Build history of the part. All positions in model axes, mm. Give positions to 0.01 mm unless a question says otherwise; leave off trailing zeros. Write each loop counter-clockwise with the first axis right and the second up, starting at its lowest first coordinate (ties: lowest second). Pieces come first, ordered by that corner, then holes.
from build123d import *

# Parameters (mm, degrees)
SKETCH1_R           = 1.575
SKETCH1_R_2         = 1.5
BOSS_EXTRUDE1_DEPTH = 3
FILLET1_R           = 5
SKETCH2_R           = 1.6
SKETCH2_R_2         = 1.5
SKETCH2_W           = 1
SKETCH2_H           = 3
SKETCH2_W_2         = 1.255583802
CUT_EXTRUDE1_DEPTH  = 3


with BuildPart() as part:
    # Sketch1 → Boss-Extrude1 (new body)
    with BuildSketch(Plane(origin=(0, 0, 0), x_dir=(1, 0, 0), z_dir=(0, 1, 0))):
        Polygon((30.311923219, 82.53968254), (-139.688076781, 82.53968254), (-139.688076781, -117.46031746), (30.311923219, -117.46031746), (30.311923219, -77.46031746), (110.311923219, -77.46031746), (110.311923219, 42.53968254), (30.311923219, 42.53968254), align=None)
        with Locations(Location((-126.688076781, -17.46031746, 0), (0, 0, 270))):
            Circle(SKETCH1_R, mode=Mode.SUBTRACT)
        with Locations(Location((-116.188076781, -11.398139634, 0), (0, 0, 270))):
            Circle(SKETCH1_R, mode=Mode.SUBTRACT)
        with Locations(Location((-116.188076781, -23.522495287, 0), (0, 0, 270))):
            Circle(SKETCH1_R, mode=Mode.SUBTRACT)
        with Locations(Location((-129.688076781, 72.53968254, 0), (0, 0, 270))):
            Circle(SKETCH1_R_2, mode=Mode.SUBTRACT)
        with Locations(Location((20.311923219, 72.53968254, 0), (0, 0, 270))):
            Circle(SKETCH1_R_2, mode=Mode.SUBTRACT)
        with Locations(Location((81.311923219, 35.03968254, 0), (0, 0, 270))):
            Circle(SKETCH1_R_2, mode=Mode.SUBTRACT)
        with Locations(Location((81.311923219, 25.03968254, 0), (0, 0, 270))):
            Circle(SKETCH1_R_2, mode=Mode.SUBTRACT)
        with Locations(Location((81.311923219, 15.03968254, 0), (0, 0, 270))):
            Circle(SKETCH1_R_2, mode=Mode.SUBTRACT)
        with Locations(Location((81.311923219, 5.03968254, 0), (0, 0, 270))):
            Circle(SKETCH1_R_2, mode=Mode.SUBTRACT)
        with Locations(Location((81.311923219, -4.96031746, 0), (0, 0, 270))):
            Circle(SKETCH1_R_2, mode=Mode.SUBTRACT)
        with Locations(Location((59.311923219, -4.96031746, 0), (0, 0, 90))):
            Circle(SKETCH1_R_2, mode=Mode.SUBTRACT)
        with Locations(Location((59.311923219, 5.03968254, 0), (0, 0, 90))):
            Circle(SKETCH1_R_2, mode=Mode.SUBTRACT)
        with Locations(Location((59.311923219, 15.03968254, 0), (0, 0, 90))):
            Circle(SKETCH1_R_2, mode=Mode.SUBTRACT)
        with Locations(Location((59.311923219, 25.03968254, 0), (0, 0, 90))):
            Circle(SKETCH1_R_2, mode=Mode.SUBTRACT)
        with Locations(Location((59.311923219, 35.03968254, 0), (0, 0, 90))):
            Circle(SKETCH1_R_2, mode=Mode.SUBTRACT)
        with Locations(Location((81.311923219, -69.96031746, 0), (0, 0, 90))):
            Circle(SKETCH1_R_2, mode=Mode.SUBTRACT)
        with Locations(Location((81.311923219, -59.96031746, 0), (0, 0, 90))):
            Circle(SKETCH1_R_2, mode=Mode.SUBTRACT)
        with Locations(Location((81.311923219, -49.96031746, 0), (0, 0, 90))):
            Circle(SKETCH1_R_2, mode=Mode.SUBTRACT)
        with Locations(Location((81.311923219, -39.96031746, 0), (0, 0, 90))):
            Circle(SKETCH1_R_2, mode=Mode.SUBTRACT)
        with Locations(Location((81.311923219, -29.96031746, 0), (0, 0, 90))):
            Circle(SKETCH1_R_2, mode=Mode.SUBTRACT)
        with Locations(Location((59.311923219, -29.96031746, 0), (0, 0, 270))):
            Circle(SKETCH1_R_2, mode=Mode.SUBTRACT)
        with Locations(Location((59.311923219, -39.96031746, 0), (0, 0, 270))):
            Circle(SKETCH1_R_2, mode=Mode.SUBTRACT)
        with Locations(Location((59.311923219, -49.96031746, 0), (0, 0, 270))):
            Circle(SKETCH1_R_2, mode=Mode.SUBTRACT)
        with Locations(Location((59.311923219, -59.96031746, 0), (0, 0, 270))):
            Circle(SKETCH1_R_2, mode=Mode.SUBTRACT)
        with Locations(Location((59.311923219, -69.96031746, 0), (0, 0, 270))):
            Circle(SKETCH1_R_2, mode=Mode.SUBTRACT)
        with Locations(Location((100.311923219, 32.53968254, 0), (0, 0, 270))):
            Circle(SKETCH1_R_2, mode=Mode.SUBTRACT)
        with Locations(Location((40.311923219, 32.53968254, 0), (0, 0, 90))):
            Circle(SKETCH1_R_2, mode=Mode.SUBTRACT)
        with Locations(Location((100.311923219, -67.46031746, 0), (0, 0, 90))):
            Circle(SKETCH1_R_2, mode=Mode.SUBTRACT)
        with Locations(Location((40.311923219, -67.46031746, 0), (0, 0, 270))):
            Circle(SKETCH1_R_2, mode=Mode.SUBTRACT)
        with Locations(Location((20.311923219, -107.46031746, 0), (0, 0, 90))):
            Circle(SKETCH1_R_2, mode=Mode.SUBTRACT)
        with Locations(Location((-129.688076781, -107.46031746, 0), (0, 0, 90))):
            Circle(SKETCH1_R_2, mode=Mode.SUBTRACT)
    extrude(amount=BOSS_EXTRUDE1_DEPTH)

    # Fillet1
    fillet1_edges = [part.edges().sort_by_distance(p)[0] for p in [
        (-139.688076781, 1.5, -82.53968254),
        (30.311923219, 1.5, -82.53968254),
        (30.311923219, 1.5, -42.53968254),
        (110.311923219, 1.5, -42.53968254),
        (110.311923219, 1.5, 77.46031746),
        (30.311923219, 1.5, 77.46031746),
        (30.311923219, 1.5, 117.46031746),
        (-139.688076781, 1.5, 117.46031746),
    ]]
    fillet(fillet1_edges, radius=FILLET1_R)

    # Sketch2 → Cut-Extrude1 (cut)
    with BuildSketch(Plane(origin=(0, 3, 0), x_dir=(1, 0, 0), z_dir=(0, 1, 0))):
        with Locations(Location((101.931923219, -39.05031746, 0), (0, 0, 270))):
            Circle(SKETCH2_R)
        with Locations(Location((94.311923219, 4.12968254, 0), (0, 0, 270))):
            Circle(SKETCH2_R)
        with Locations(Location((41.101923219, -7.85531746, 0), (0, 0, 270))):
            Circle(SKETCH2_R)
        with Locations(Location((41.101923219, 11.35468254, 0), (0, 0, 270))):
            Circle(SKETCH2_R)
        with Locations(Location((41.101923219, -46.27531746, 0), (0, 0, 270))):
            Circle(SKETCH2_R)
        with Locations(Location((41.101923219, -27.06531746, 0), (0, 0, 270))):
            Circle(SKETCH2_R)
        with Locations(Location((-14.518076781, -7.85531746, 0), (0, 0, 270))):
            Circle(SKETCH2_R)
        with Locations(Location((-14.518076781, 11.35468254, 0), (0, 0, 270))):
            Circle(SKETCH2_R)
        with Locations(Location((-14.518076781, -27.06531746, 0), (0, 0, 270))):
            Circle(SKETCH2_R)
        with Locations(Location((-14.518076781, -46.27531746, 0), (0, 0, 270))):
            Circle(SKETCH2_R)
        with Locations(Location((-49.062510974, -52.38531746, 0), (0, 0, 270))):
            Circle(SKETCH2_R_2)
        with Locations(Location((-49.062510974, 17.46468254, 0), (0, 0, 270))):
            Circle(SKETCH2_R_2)
        with Locations(Location((70.311923219, -51.21031746, 0), (0, 0, 270))):
            Circle(SKETCH2_R_2)
        with Locations(Location((70.311923219, 16.28968254, 0), (0, 0, 270))):
            Circle(SKETCH2_R_2)
        with Locations(Location((27.931923219, 14.35968254, 0), (0, 0, 270))):
            Circle(SKETCH2_R)
        with Locations(Location((20.311923219, 57.53968254, 0), (0, 0, 270))):
            Circle(SKETCH2_R)
        with Locations((49.311923219, -7.85531746)):
            Rectangle(SKETCH2_W, SKETCH2_H)
        with Locations((49.311923219, -27.06531746)):
            Rectangle(SKETCH2_W, SKETCH2_H)
        with Locations((49.311923219, -46.27531746)):
            Rectangle(SKETCH2_W_2, SKETCH2_H)
        with Locations((49.311923219, 11.35468254)):
            Rectangle(SKETCH2_W_2, SKETCH2_H)
        with Locations((-22.728076781, 11.35468254)):
            Rectangle(SKETCH2_W_2, SKETCH2_H)
        with Locations((-22.728076781, -7.85531746)):
            Rectangle(SKETCH2_W, SKETCH2_H)
        with Locations((-22.728076781, -27.06531746)):
            Rectangle(SKETCH2_W, SKETCH2_H)
        with Locations((-22.728076781, -46.27531746)):
            Rectangle(SKETCH2_W_2, SKETCH2_H)
    extrude(amount=-CUT_EXTRUDE1_DEPTH, mode=Mode.SUBTRACT)


solid = part.part
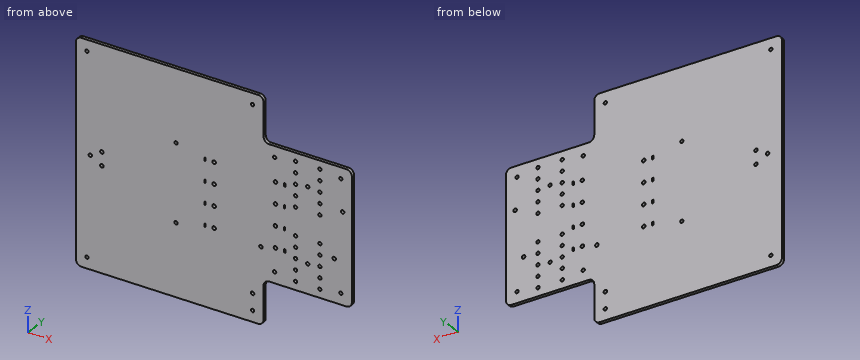
1. Saw through at B-B on y = 1. Count the separate pieces of the cut face and the enclosed holes in it, plus the area to 3 significant figures.
2. Drop flat-ended pins along their axis: pin 1 (1.1 mm diameter, centred on x = 49.5, y = 1.5, fed in from -Z); pin 2 (0.8 mm diameter, centred on x = 49.5, y = 1, fed in from +Z). Give the stop position or say it passes through.
3. Drill centre lines: line 1 along X through (y, z) = (1.8, 70.5); line 2 along X through (y, z) = (1.9, 47.5); line 3 along Z through (x, y) = (-115, 1.4). Where is each one in solid material? Low to high.
4. Saw through at A-A on z = -63. Give the cut face in (x, y).
Outcome:
1. separate pieces: 1
1. enclosed holes: 55
1. area: 43,200 mm2
2. pin 1: stops at z = -42.54
2. pin 2: stops at z = 77.46
3. line 1: x = -139.69 to 57.91, 60.71 to 79.91, 82.71 to 110.31
3. line 2: x = -139.69 to -23.36, -22.1 to -15.55, -13.49 to 40.07, 42.13 to 48.68, 49.94 to 110.31
3. line 3: z = -82.54 to 10.36, 12.43 to 22.49, 24.56 to 117.46
4. outline: (-139.69, 0) - (30.31, 0) - (30.31, 3) - (-139.69, 3) - close
